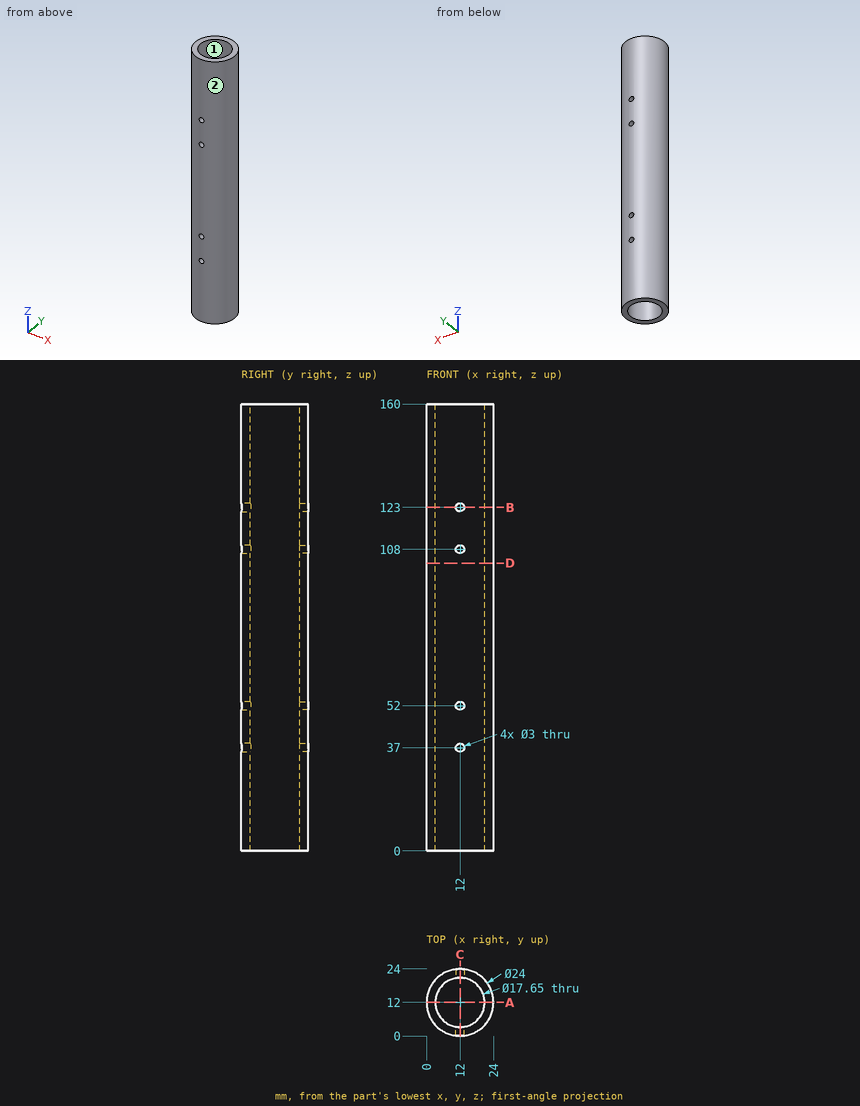
Could you check a few things on this drawing? It's one solid part, dimensions in mm from its lowest x, y, z. Round coordinates to 2 decimals unless told otherwise and drop trailing zeros. Order: outer loops, then holes, each group sorted by start corner. A loop starts at its lowest first (then second) coordinate and runs counter-clockwise, first axis right, second up.
(1) Imagine slicing it at C-C (x = 12). Count the separate pieces of the cut face and the enclosed holes in it, plus the area to 3 significant figures.
Response values:
separate pieces: 10
enclosed holes: 0
area: 940 mm2
(2) Please list where these lines run through material, in increasing order: line 1 along Y through (x, z) = (12, 87) (3 decimals); line 2 along X through (y, z) = (1.45, 123); line 3 along Y through (x, z) = (14.5, 26).
Response values:
line 1: y = 0 to 3.175, 20.825 to 24
line 2: x = 6.28 to 10.5, 13.5 to 17.72
line 3: y = 0.26 to 3.54, 20.46 to 23.74
(3) I'm going to push flat-ended pins straight in: pin 1 (1 mm diameter, centred on x = 9, z = 93.5, fed in from -Y); pin 2 (5 mm diameter, centred on y = 15, z = 47.5, fed in from +X); pin 3 (1.5 mm diameter, centred on x = 7.5, z = 112.5, fed in from -Y). Where does each tip first touch, or does it pass through?
Response values:
pin 1: stops at y = 0.26
pin 2: stops at x = 23.99
pin 3: stops at y = 0.6
(4) If we mould it in two halves opening along X, with no side actions, what happens to the marked faces 1 and 2? For each: released by +X, released by -X, zero draft, split by the parting line, or undercut.
Response values:
face 1: undercut
face 2: split by the parting line
(5) Imagine slicing it at B-B (z = 123). Write out the boundary of the cut face in (x, y) (3 decimals).
Response values:
outline: (10.5, 0.094) - (10.5, 3.303) arc R8.825 cw to (10.5, 20.697) - (10.5, 23.906) arc R12 ccw to start; (13.5, 0.094) arc R12 ccw to (13.5, 23.906) - (13.5, 20.697) arc R8.825 cw to (13.5, 3.303) - close
(6) Imagine slicing it at A-A (y = 12). Write out the boundary of the cut face in (x, z) (3 decimals), plus the area to 3 significant figures.
Response values:
outline: (0, 0) - (3.175, 0) - (3.175, 160) - (0, 160) - close; (20.825, 0) - (24, 0) - (24, 160) - (20.825, 160) - close
area: 1,020 mm2
(7) Imagine slicing it at D-D (z = 103). Write out the boundary of the cut face in (x, y) (3 decimals), plus the area to 3 significant figures.
Response values:
outline: circle Ø24 at (12, 12); hole circle Ø17.65 at (12, 12)
area: 208 mm2
